from build123d import *

# Parameters (mm, degrees)
BOSS_EXTRU_1_DEPTH      = 15
ESQUISSE3_R             = 6.25
ESQUISSE3_R_2           = 1.55
ENL_V_MAT_EXTRU_1_DEPTH = 54.528403675
ESQUISSE4_R             = 1.35
ENL_V_MAT_EXTRU_2_DEPTH = 78.679083414


with BuildPart() as part:
    # Esquisse1 → Boss.-Extru.1 (new, symmetric)
    with BuildSketch(Plane.XY):
        Polygon((-25, 39.8), (25, 39.8), (32.5, 32.875544179), (32.5, 0), (30.5, 0), (30.5, 32), (24.217917895, 37.8), (-24.217917895, 37.8), (-30.5, 32), (-30.5, 0), (-32.5, 0), (-32.5, 32.875544179), align=None)
    extrude(amount=BOSS_EXTRU_1_DEPTH, both=True)

    # Esquisse3 → Enlèv. mat.-Extru.1 (cut, through all)
    with BuildSketch(Plane(origin=(0, 39.8, 0), x_dir=(1, 0, 0), z_dir=(0, 1, 0))):
        with Locations(Location((0, 0, 0), (0, 0, 270))):
            Circle(ESQUISSE3_R)
        with Locations(Location((-8.485281374, 8.485281374, 0), (0, 0, 270))):
            Circle(ESQUISSE3_R_2)
        with Locations(Location((-8.485281374, -8.485281374, 0), (0, 0, 270))):
            Circle(ESQUISSE3_R_2)
        with Locations(Location((8.485281374, -8.485281374, 0), (0, 0, 270))):
            Circle(ESQUISSE3_R_2)
        with Locations(Location((8.485281374, 8.485281374, 0), (0, 0, 270))):
            Circle(ESQUISSE3_R_2)
        with Locations(Location((20, 10.5, 0), (0, 0, 270))):
            Circle(ESQUISSE3_R_2)
        with Locations(Location((-20, 10.5, 0), (0, 0, 270))):
            Circle(ESQUISSE3_R_2)
        with Locations(Location((20, -10.5, 0), (0, 0, 270))):
            Circle(ESQUISSE3_R_2)
        with Locations(Location((-20, -10.5, 0), (0, 0, 270))):
            Circle(ESQUISSE3_R_2)
    extrude(amount=-ENL_V_MAT_EXTRU_1_DEPTH, mode=Mode.SUBTRACT)

    # Esquisse4 → Enlèv. mat.-Extru.2 (cut, through all)
    with BuildSketch(Plane(origin=(32.5, 0, 0), x_dir=(0, 0, -1), z_dir=(1, 0, 0))):
        with Locations((-12, 4.8)):
            Circle(ESQUISSE4_R)
        with Locations((0, 16.8)):
            Circle(ESQUISSE4_R)
        with Locations((-8.485281374, 13.285281374)):
            Circle(ESQUISSE4_R)
        with Locations(Location((12, 4.8, 0), (0, 0, 180))):
            Circle(ESQUISSE4_R)
        with Locations(Location((8.485281374, 13.285281374, 0), (0, 0, 180))):
            Circle(ESQUISSE4_R)
        with BuildLine():
            Line((-6.2, 0), (-6.2, 4.8))
            ThreePointArc((-6.2, 4.8), (0, 11), (6.2, 4.8))
            Line((6.2, 4.8), (6.2, 0))
            Line((6.2, 0), (-6.2, 0))
        make_face()
    extrude(amount=-ENL_V_MAT_EXTRU_2_DEPTH, mode=Mode.SUBTRACT)


solid = part.part
Geometry: final body of the model. Coordinates: model frame, mm. A direction names the side the tool comes from. Coordinates: 2 decimals unless noted, no trailing zeros. Order: outer loops, then holes, each group sorted by start corner. A loop starts at its lowest first (then second) coordinate and runs counter-clockwise, first axis right, second up.
(1) Access query for faces 1 (the face through (-31.486, 11.967, 8.778)), 2 (the face through (-31, 2, -6.2)). Directions: +Z, -Z, +X, -X, +Y, -Y. A direction counts if a zero-diameter tool reaches every point of the face in a straight line with its end or side. Return the directions, or none.
(2) Section query D-D (z = 3.5). Return the cut outline in (x, y), plus the area to 3 significant figures.
(3) Material intervals for probe 1 along X at (y, z) = (24.5, -11.25); probe 2 along Y at (x, z) = (19, -4.5); probe 3 along Y at (x, z) = (31.4, -12), sorted ascending.
(4) First-contact query: pin 1 (10 mm diameter, centred on x = -5.5, z = -7.5, fed in from -Y); pin 2 (2.5 mm diameter, centred on x = -20, z = 10.5, fed in from +Y). Flat tips, straight axial feed; report the tip coordinate or a pass-through.
(5) Section query B-B (y = 19). Return the cut outline in (x, z).
(6) Section query A-A (z = 0). Return the cut outline in (x, y), plus the area to 3 significant figures.
(7) Draft query along Y for faces 3 (the face through (8.951, 38.814, 9.964)), 4 (the face through (-31.49, 6, -11.38)), 5 (the face through (28.698, 36.386, 0.21)). Return one class per face: pulls with the +Y half, pulls with the -Y half, needs draft (parallel to the pull), parting line crosses it, or undercut.
(8) Section query C-C (x = 20). Return the cut outline in (y, z).
Solution:
1. face 1: +X, -X
1. face 2: +X, -X, -Y
2. outline: (-32.5, 9.92) - (-30.5, 9.92) - (-30.5, 32) - (-24.22, 37.8) - (-5.18, 37.8) - (-5.18, 39.8) - (-25, 39.8) - (-32.5, 32.88) - close; (5.18, 37.8) - (24.22, 37.8) - (30.5, 32) - (30.5, 9.92) - (32.5, 9.92) - (32.5, 32.88) - (25, 39.8) - (5.18, 39.8) - close
2. area: 205 mm2
3. probe 1: x = -32.5 to -30.5, 30.5 to 32.5
3. probe 2: y = 37.8 to 39.8
3. probe 3: y = 0 to 3.45, 6.15 to 33.89
4. pin 1: stops at y = 37.8
4. pin 2: passes through
5. outline: (-32.5, -15) - (-30.5, -15) - (-30.5, 15) - (-32.5, 15) - close; (30.5, -15) - (32.5, -15) - (32.5, 15) - (30.5, 15) - close
6. outline: (-32.5, 11) - (-30.5, 11) - (-30.5, 15.45) - (-32.5, 15.45) - close; (-32.5, 18.15) - (-30.5, 18.15) - (-30.5, 32) - (-24.22, 37.8) - (-6.25, 37.8) - (-6.25, 39.8) - (-25, 39.8) - (-32.5, 32.88) - close; (6.25, 37.8) - (24.22, 37.8) - (30.5, 32) - (30.5, 18.15) - (32.5, 18.15) - (32.5, 32.88) - (25, 39.8) - (6.25, 39.8) - close; (30.5, 11) - (32.5, 11) - (32.5, 15.45) - (30.5, 15.45) - close
6. area: 186 mm2
7. face 3: needs draft
7. face 4: undercut
7. face 5: pulls with the +Y half
8. outline: (37.8, -15) - (39.8, -15) - (39.8, -12.05) - (37.8, -12.05) - close; (37.8, -8.95) - (39.8, -8.95) - (39.8, 8.95) - (37.8, 8.95) - close; (37.8, 12.05) - (39.8, 12.05) - (39.8, 15) - (37.8, 15) - close
